Source: CAD feature listing. Evaluate the final solid. Frame: model axes, mm. Face numbers are marked on the shaded views. A direction names the side the tool comes from. Give positions to 0.01 mm unless a question says otherwise; leave off trailing zeros. Loops run counter-clockwise (first coordinate to the right, second up) from the corner with the lowest first, then second, coordinate; pieces in that order, holes last. Notation, with made-up numbers: M 81,14 L 95,14 A13 cw 95,19 Z; hole C -33,13 d10. An arc over 180 degrees is marked long. Put each result on its own line as item: value.
from build123d import *

# Parameters (mm, degrees)
F1_DEPTH = 4.5
F2_R     = 4.5
F3_R     = 3
F4_R     = 0.5
F5_R     = 6


with BuildPart() as f1:
    # F0 (on Top) → F1 (new body)
    with BuildSketch(Plane.XY):
        with BuildLine():
            ThreePointArc((9.564743, -1.89161), (0, 9.75), (-9.564743, -1.89161))
            Line((-9.564743, -1.89161), (-8.95, -5))
            Line((-8.95, -5), (-23.5, -23.438322))
            Line((-23.5, -23.438322), (-23.5, -33))
            Line((-23.5, -33), (23.5, -33))
            Line((23.5, -33), (23.5, -23.438322))
            Line((23.5, -23.438322), (8.95, -5))
            Line((8.95, -5), (9.564743, -1.89161))
        make_face()
        with BuildLine():
            ThreePointArc((-4.45, -2.785678), (0, 5.25), (4.45, -2.785678))
            Line((4.45, -2.785678), (4.45, -6.561678))
            Line((4.45, -6.561678), (19, -25))
            Line((19, -25), (19, -28.5))
            Line((19, -28.5), (-19, -28.5))
            Line((-19, -28.5), (-19, -25))
            Line((-19, -25), (-4.45, -6.561678))
            Line((-4.45, -6.561678), (-4.45, -2.785678))
        make_face(mode=Mode.SUBTRACT)
    extrude(amount=F1_DEPTH)

    # F2
    f2_edges = [f1.edges().sort_by_distance(p)[0] for p in [
        (-19, -25, 2.25),
        (19, -25, 2.25),
        (-23.5, -33, 2.25),
        (23.5, -33, 2.25),
    ]]
    fillet(f2_edges, radius=F2_R)

    # F3
    f3_edges = [f1.edges().sort_by_distance(p)[0] for p in [
        (-8.95, -5, 2.25),
        (8.95, -5, 2.25),
        (23.5, -23.438322, 2.25),
        (-23.5, -23.438322, 2.25),
    ]]
    fillet(f3_edges, radius=F3_R)

    # F4
    f4_edges = [f1.edges().sort_by_distance(p)[0] for p in [
        (-19, -28.5, 2.25),
        (19, -28.5, 2.25),
    ]]
    fillet(f4_edges, radius=F4_R)

    # F5
    f5_edges = [f1.edges().sort_by_distance(p)[0] for p in [
        (4.45, -6.561678, 2.25),
        (-4.45, -6.561678, 2.25),
        (4.45, -2.785678, 2.25),
        (-4.45, -2.785678, 2.25),
    ]]
    fillet(f5_edges, radius=F5_R)


solid = f1.part
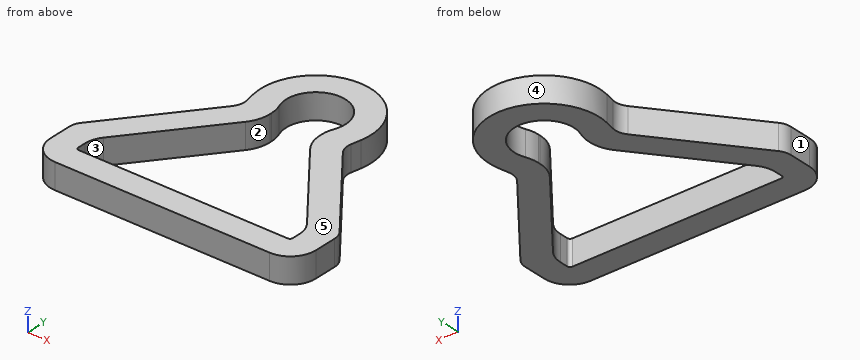
1. Draft query along X for the marked faces 3, 4 and 5. Return one class per face: pulls with the +X half, pulls with the -X half, needs draft (parallel to the pull), parting line crosses it, or undercut.
Found:
face 3: undercut
face 4: parting line crosses it
face 5: needs draft
2. Access query for the marked faces 1 and 2. Directions: +Z, -Z, +X, -X, +Y, -Y. A direction counts if a zero-diameter tool reaches every point of the face in a straight line with its end or side. Return the directions, or none.
Found:
face 1: +Z, -Z, -X, +Y, -Y
face 2: +Z, -Z
3. Material intervals for line 1 (X direction, y = 0, z = 3.25); line 2 (X direction, y = -2, z = 0.5); line 3 (Y direction, x = -13, z = 0.8), sorted ascending. Write a range as from..to.
Found:
line 1: -9.75..-5.25, 5.25..9.75
line 2: -9.54..-4.85, 4.85..9.54
line 3: -33..-28.5, -17.4..-10.13
4. Section query B-B (y = 0). Output: boundary loops of the cut face in (x, z), plus the area to 3 significant figures.
Found:
outline: M -9.75,0 L -5.25,0 L -5.25,4.5 L -9.75,4.5 Z; M 5.25,0 L 9.75,0 L 9.75,4.5 L 5.25,4.5 Z
area: 40.5 mm^2
5. Contact query for flat-ended pins moving along their axis: P1, Ø2, axis at x = 8, z = 3.5, coming from the +Y side; P2, Ø1.5, axis at x = 16.5, z = 2, coming from the +Y side. Output: stop coordinate, or through.
Found:
P1: y = 6.79
P2: y = -13.62
6. Section query A-A (x = 0). Output: boundary loops of the cut face in (y, z), plus the area to 3 significant figures.
Found:
outline: M -33,0 L -28.5,0 L -28.5,4.5 L -33,4.5 Z; M 5.25,0 L 9.75,0 L 9.75,4.5 L 5.25,4.5 Z
area: 40.5 mm^2
